from build123d import *

# Parameters (mm, degrees)
SKETCH2_R           = 4.05
BOSS_EXTRUDE1_DEPTH = 2
BOSS_EXTRUDE2_DEPTH = 40
BOSS_EXTRUDE3_DEPTH = 5
BOSS_EXTRUDE4_DEPTH = 2
SKETCH10_R          = 2.5
BOSS_EXTRUDE5_DEPTH = 7
DOME1_FACE_RADIUS   = 2.5
DOME1_HEIGHT        = 1
SKETCH12_R          = 2.5
BOSS_EXTRUDE6_DEPTH = 0.75
DOME2_FACE_RADIUS   = 2.5
DOME2_HEIGHT        = 1


with BuildPart() as part:
    # Sketch2 → Boss-Extrude1 (new body)
    with BuildSketch(Plane.XY):
        with BuildLine():
            Line((-100, 0), (-100, -100))
            Line((-100, -100), (100, -100))
            Line((100, -100), (100, 0))
            ThreePointArc((100, 0), (0, 100), (-100, 0))
        make_face()
        Circle(SKETCH2_R, mode=Mode.SUBTRACT)
        with BuildLine():
            Line((6.470476128, 24.148145657), (10.352761804, 38.637033052))
            ThreePointArc((10.352761804, 38.637033052), (0, 40), (-10.352761804, 38.637033052))
            Line((-10.352761804, 38.637033052), (-6.470476128, 24.148145657))
            ThreePointArc((-6.470476128, 24.148145657), (0, 25), (6.470476128, 24.148145657))
        make_face(mode=Mode.SUBTRACT)
        with BuildLine():
            Line((14.235047481, 53.125920446), (18.117333157, 67.61480784))
            ThreePointArc((18.117333157, 67.61480784), (0, 70), (-18.117333157, 67.61480784))
            Line((-18.117333157, 67.61480784), (-14.235047481, 53.125920446))
            ThreePointArc((-14.235047481, 53.125920446), (0, 55), (14.235047481, 53.125920446))
        make_face(mode=Mode.SUBTRACT)
        with BuildLine():
            Line((-20, 34.641016151), (-27.5, 47.631397208))
            ThreePointArc((-27.5, 47.631397208), (-38.890872965, 38.890872965), (-47.631397208, 27.5))
            Line((-47.631397208, 27.5), (-34.641016151, 20))
            ThreePointArc((-34.641016151, 20), (-28.284271247, 28.284271247), (-20, 34.641016151))
        make_face(mode=Mode.SUBTRACT)
        with BuildLine():
            Line((-35, 60.621778265), (-42.5, 73.612159322))
            ThreePointArc((-42.5, 73.612159322), (-60.104076401, 60.104076401), (-73.612159322, 42.5))
            Line((-73.612159322, 42.5), (-60.621778265, 35))
            ThreePointArc((-60.621778265, 35), (-49.497474683, 49.497474683), (-35, 60.621778265))
        make_face(mode=Mode.SUBTRACT)
        with BuildLine():
            Line((42.5, 73.612159322), (35, 60.621778265))
            ThreePointArc((35, 60.621778265), (49.497474683, 49.497474683), (60.621778265, 35))
            Line((60.621778265, 35), (73.612159322, 42.5))
            ThreePointArc((73.612159322, 42.5), (60.104076401, 60.104076401), (42.5, 73.612159322))
        make_face(mode=Mode.SUBTRACT)
        with BuildLine():
            Line((27.5, 47.631397208), (20, 34.641016151))
            ThreePointArc((20, 34.641016151), (28.284271247, 28.284271247), (34.641016151, 20))
            Line((34.641016151, 20), (47.631397208, 27.5))
            ThreePointArc((47.631397208, 27.5), (38.890872965, 38.890872965), (27.5, 47.631397208))
        make_face(mode=Mode.SUBTRACT)
        with BuildLine():
            Line((24.148145657, -6.470476128), (38.637033052, -10.352761804))
            ThreePointArc((38.637033052, -10.352761804), (40, 0), (38.637033052, 10.352761804))
            Line((38.637033052, 10.352761804), (24.148145657, 6.470476128))
            ThreePointArc((24.148145657, 6.470476128), (25, 0), (24.148145657, -6.470476128))
        make_face(mode=Mode.SUBTRACT)
        with BuildLine():
            Line((53.125920446, -14.235047481), (67.61480784, -18.117333157))
            ThreePointArc((67.61480784, -18.117333157), (70, 0), (67.61480784, 18.117333157))
            Line((67.61480784, 18.117333157), (53.125920446, 14.235047481))
            ThreePointArc((53.125920446, 14.235047481), (55, 0), (53.125920446, -14.235047481))
        make_face(mode=Mode.SUBTRACT)
        with BuildLine():
            Line((73.612159322, -42.5), (60.621778265, -35))
            ThreePointArc((60.621778265, -35), (49.497474683, -49.497474683), (35, -60.621778265))
            Line((35, -60.621778265), (42.5, -73.612159322))
            ThreePointArc((42.5, -73.612159322), (60.104076401, -60.104076401), (73.612159322, -42.5))
        make_face(mode=Mode.SUBTRACT)
        with BuildLine():
            Line((47.631397208, -27.5), (34.641016151, -20))
            ThreePointArc((34.641016151, -20), (28.284271247, -28.284271247), (20, -34.641016151))
            Line((20, -34.641016151), (27.5, -47.631397208))
            ThreePointArc((27.5, -47.631397208), (38.890872965, -38.890872965), (47.631397208, -27.5))
        make_face(mode=Mode.SUBTRACT)
        with BuildLine():
            Line((-6.470476128, -24.148145657), (-10.352761804, -38.637033052))
            ThreePointArc((-10.352761804, -38.637033052), (0, -40), (10.352761804, -38.637033052))
            Line((10.352761804, -38.637033052), (6.470476128, -24.148145657))
            ThreePointArc((6.470476128, -24.148145657), (0, -25), (-6.470476128, -24.148145657))
        make_face(mode=Mode.SUBTRACT)
        with BuildLine():
            Line((-14.235047481, -53.125920446), (-18.117333157, -67.61480784))
            ThreePointArc((-18.117333157, -67.61480784), (0, -70), (18.117333157, -67.61480784))
            Line((18.117333157, -67.61480784), (14.235047481, -53.125920446))
            ThreePointArc((14.235047481, -53.125920446), (0, -55), (-14.235047481, -53.125920446))
        make_face(mode=Mode.SUBTRACT)
        with BuildLine():
            Line((-42.5, -73.612159322), (-35, -60.621778265))
            ThreePointArc((-35, -60.621778265), (-49.497474683, -49.497474683), (-60.621778265, -35))
            Line((-60.621778265, -35), (-73.612159322, -42.5))
            ThreePointArc((-73.612159322, -42.5), (-60.104076401, -60.104076401), (-42.5, -73.612159322))
        make_face(mode=Mode.SUBTRACT)
        with BuildLine():
            Line((-27.5, -47.631397208), (-20, -34.641016151))
            ThreePointArc((-20, -34.641016151), (-28.284271247, -28.284271247), (-34.641016151, -20))
            Line((-34.641016151, -20), (-47.631397208, -27.5))
            ThreePointArc((-47.631397208, -27.5), (-38.890872965, -38.890872965), (-27.5, -47.631397208))
        make_face(mode=Mode.SUBTRACT)
        with BuildLine():
            Line((-24.148145657, 6.470476128), (-38.637033052, 10.352761804))
            ThreePointArc((-38.637033052, 10.352761804), (-40, 0), (-38.637033052, -10.352761804))
            Line((-38.637033052, -10.352761804), (-24.148145657, -6.470476128))
            ThreePointArc((-24.148145657, -6.470476128), (-25, 0), (-24.148145657, 6.470476128))
        make_face(mode=Mode.SUBTRACT)
        with BuildLine():
            Line((-53.125920446, 14.235047481), (-67.61480784, 18.117333157))
            ThreePointArc((-67.61480784, 18.117333157), (-70, 0), (-67.61480784, -18.117333157))
            Line((-67.61480784, -18.117333157), (-53.125920446, -14.235047481))
            ThreePointArc((-53.125920446, -14.235047481), (-55, 0), (-53.125920446, 14.235047481))
        make_face(mode=Mode.SUBTRACT)
    extrude(amount=BOSS_EXTRUDE1_DEPTH)

    # Sketch4 → Boss-Extrude2 (add)
    with BuildSketch(Plane(origin=(0, 0, 0), x_dir=(-1, 0, 0), z_dir=(0, 0, -1))):
        Polygon((-70.814, -63.74), (-48.634, -63.74), (-48.634, -58.54), (-45.574, -58.54), (-45.574, -36.410509339), (-41.222261094, -36.410509339), (-41.222261094, -63.74), (-41.222261094, -66.24), (-76.222261094, -66.24), (-81.222261094, -66.24), (-81.222261094, 0.239543082), (-78.722261094, 0.239543082), (-78.722261094, -36.363042073), (-73.874, -36.363042073), (-73.874, -58.54), (-70.814, -58.54), align=None)
        Polygon((81.222261094, -66.24), (76.222261094, -66.24), (41.222261094, -66.24), (41.222261094, -63.74), (41.222261094, -36.410509339), (45.574, -36.410509339), (45.574, -58.54), (48.634, -58.54), (48.634, -63.74), (70.814, -63.74), (70.814, -58.54), (73.874, -58.54), (73.874, -36.363042073), (78.722261094, -36.363042073), (78.722261094, 0.239543082), (81.222261094, 0.239543082), align=None)
    extrude(amount=BOSS_EXTRUDE2_DEPTH)

    # Sketch7 → Boss-Extrude3 (add, symmetric)
    with BuildSketch(Plane(origin=(63, 0, 0), x_dir=(0, 0, -1), z_dir=(1, 0, 0))):
        Polygon((0, -86.447259422), (35, -66.24), (26.86565258, -66.24), (0, -81.750891749), align=None)
    boss_extrude3 = extrude(amount=BOSS_EXTRUDE3_DEPTH, both=True)

    # Mirror1: Boss-Extrude3 across plane
    add(boss_extrude3.mirror(Plane(origin=(0, 0, 0), x_dir=(0, 0, 1), z_dir=(1, 0, 0))))


with BuildPart() as boss_extrude4_tool:
    # Sketch8 → Boss-Extrude4 (new body)
    with BuildSketch(Plane.XY.offset(2)):
        with BuildLine():
            Line((-54.94315244, 2.5), (-69.955342898, 2.5))
            add(Edge.make_bspline(
                [(-69.955342898, 2.5), (-70.044657102, 0), (-69.955342898, -2.5)],
                knots=[0, 0, 0, 1, 1, 1], degree=2))
            Line((-69.955342898, -2.5), (-54.94315244, -2.5))
            add(Edge.make_bspline(
                [(-54.94315244, 2.5), (-55.05684756, 0), (-54.94315244, -2.5)],
                knots=[0, 0, 0, 1, 1, 1], degree=2))
        make_face()
        with BuildLine():
            Line((-2.5, 54.94315244), (-2.5, 69.955342898))
            add(Edge.make_bspline(
                [(2.5, 69.955342898), (0, 70.044657102), (-2.5, 69.955342898)],
                knots=[0, 0, 0, 1, 1, 1], degree=2))
            Line((2.5, 69.955342898), (2.5, 54.94315244))
            add(Edge.make_bspline(
                [(2.5, 54.94315244), (0, 55.05684756), (-2.5, 54.94315244)],
                knots=[0, 0, 0, 1, 1, 1], degree=2))
        make_face()
        with BuildLine():
            Line((54.94315244, 2.5), (69.955342898, 2.5))
            add(Edge.make_bspline(
                [(69.955342898, -2.5), (70.044657102, 0), (69.955342898, 2.5)],
                knots=[0, 0, 0, 1, 1, 1], degree=2))
            Line((69.955342898, -2.5), (54.94315244, -2.5))
            add(Edge.make_bspline(
                [(54.94315244, -2.5), (55.05684756, 0), (54.94315244, 2.5)],
                knots=[0, 0, 0, 1, 1, 1], degree=2))
        make_face()
        with BuildLine():
            Line((2.5, -54.94315244), (2.5, -69.955342898))
            add(Edge.make_bspline(
                [(-2.5, -69.955342898), (0, -70.044657102), (2.5, -69.955342898)],
                knots=[0, 0, 0, 1, 1, 1], degree=2))
            Line((-2.5, -69.955342898), (-2.5, -54.94315244))
            add(Edge.make_bspline(
                [(-2.5, -54.94315244), (0, -55.05684756), (2.5, -54.94315244)],
                knots=[0, 0, 0, 1, 1, 1], degree=2))
        make_face()
    extrude(amount=-BOSS_EXTRUDE4_DEPTH)


with BuildPart() as part_1:
    add(part.part)


with BuildPart() as part_2:
    # Boss-Extrude4: joined with boss_extrude4_tool
    add(part_1.part.fuse(boss_extrude4_tool.part, tol=0.00001))

    # Sketch10 → Boss-Extrude5 (add)
    with BuildSketch(Plane.XY.offset(2)):
        with Locations((-59.724, 0)):
            Circle(SKETCH10_R)
    extrude(amount=-BOSS_EXTRUDE5_DEPTH)

    # Dome1: a dome of height H over a round flat face of radius A is a cap of a sphere of radius (A * A + H * H) / (2 * H)
    dome1_r = (DOME1_FACE_RADIUS * DOME1_FACE_RADIUS + DOME1_HEIGHT * DOME1_HEIGHT) / (2 * DOME1_HEIGHT)
    dome1_base = Plane((-59.724, 0, -5), z_dir=(0, 0, -1))
    with Locations(dome1_base.offset(DOME1_HEIGHT - dome1_r)):
        dome1_ball = Sphere(dome1_r, mode=Mode.PRIVATE)
    add(split(dome1_ball, bisect_by=dome1_base, keep=Keep.TOP, mode=Mode.PRIVATE))

    # Sketch12 → Boss-Extrude6 (add)
    with BuildSketch(Plane(origin=(0, 0, 0), x_dir=(-1, 0, 0), z_dir=(0, 0, -1))):
        with Locations(Location((-59.724, 0, 0), (0, 0, 270))):
            Circle(SKETCH12_R)
    extrude(amount=BOSS_EXTRUDE6_DEPTH)

    # Dome2: a dome of height H over a round flat face of radius A is a cap of a sphere of radius (A * A + H * H) / (2 * H)
    dome2_r = (DOME2_FACE_RADIUS * DOME2_FACE_RADIUS + DOME2_HEIGHT * DOME2_HEIGHT) / (2 * DOME2_HEIGHT)
    dome2_base = Plane((59.724, 0, -0.75), z_dir=(0, 0, -1))
    with Locations(dome2_base.offset(DOME2_HEIGHT - dome2_r)):
        dome2_ball = Sphere(dome2_r, mode=Mode.PRIVATE)
    add(split(dome2_ball, bisect_by=dome2_base, keep=Keep.TOP, mode=Mode.PRIVATE))


solid = part_2.part
Build history of the part. All positions in model axes, mm. A direction names the side the tool comes from. Coordinates: 2 decimals unless noted, no trailing zeros. Order: outer loops, then holes, each group sorted by start corner. A loop starts at its lowest first (then second) coordinate and runs counter-clockwise, first axis right, second up. Notation, with made-up numbers: M 17,85.5 L 43,85.5 A15 cw 43,99.5 Z; hole C 6,-33 d10. An arc over 180 degrees is marked long. One line per question, with ' | ' between items. Start each with the question number.
Q1. Flat gauge pins, fed straight in: pin 1 Ø3.5 at (x, z) = (47.5, -27) entering from +Y; pin 2 Ø1.2 at (x, z) = (80, -16) entering from +Y; pin 3 Ø1 at (x, y) = (40, 79) entering from -Z. Where does each tip first touch, or does it go through?
Q2. Saw through at B-B (y = 80.5). List the corners of the cut face in (x, z), then the cut area to 3 significant figures.
Q3. Two-plate mould, pull along Y, no slides. Class faces 1 (the face through (-81.222, -33, -20)), 2 (the face through (2.199, 99.976, 0.986)), 3 (the face through (62.165, 0.542, -0.37)): +Y half, -Y half, draft (parallel to the pull), parting line (faces both ways), or undercut.
Q4. Saw through at C-C (z = -17). Count the separate pieces of the cut face and the enclosed holes in it, then the cut area to 3 significant figures.
Q5. 3-axis set-ups, long thin cutter, end or side, ignore diameter. For faces 4 (the face through (-45.574, -47, -20)), 5 (the face through (-58, -76, -16)), 6 (the face through (48.634, -61, -20)), 7 (the face through (60.324, 59.883, 0.986)): which of +Z, -Z, +X, -X, +Y, -Y reach the whole face in a straight line?
Q6. Probe L1, parallel to X at y = -50.5, z = -21.5; L2, parallel to Y at x = 69, z = -8.5; L3, parallel to Z at x = -50, y = 48. List the from-to ranges inside material, lowest first. Write a range as from..to.
Q7. Saw through at A-A (x = 0). List the corners of the cut face in (y, z).
Check values:
1) pin 1: stops at y = -58.54 | pin 2: stops at y = 0.24 | pin 3: stops at z = 0
2) outline: M -59.33,0 L 59.33,0 L 59.33,2 L -59.33,2 Z | area: 237 mm2
3) face 1: draft | face 2: +Y half | face 3: undercut
4) separate pieces: 4 | enclosed holes: 0 | area: 1,180 mm2
5) face 4: -Z, +Y | face 5: -Z, -Y | face 6: +Z, -Z, +Y | face 7: +Z, -Z
6) L1: x = -81.22..-73.87, -45.57..-41.22, 41.22..45.57, 73.87..81.22 | L2: y = -66.24..-63.74 | L3: z = 0..2
7) outline: M -100,0 L -40,0 L -40,2 L -100,2 Z; M -25,0 L -4.05,0 L -4.05,2 L -25,2 Z; M 4.05,0 L 25,0 L 25,2 L 4.05,2 Z; M 40,0 L 100,0 L 100,2 L 40,2 Z
